```python
from build123d import *

# Parameters (mm, degrees)
BOSS_EXTRUDE5_DEPTH = 3
CUT_EXTRUDE1_DEPTH  = 9


with BuildPart() as part:
    # Sketch3 → Boss-Extrude5 (new body)
    with BuildSketch(Plane.XY):
        Polygon((-125, 125), (-125, -125), (25, -125), (35, -135), (125, -135), (125, -125), (125, 125), (125, 130), (95, 130), (90, 125), (20, 125), (15, 130), (-15, 130), (-20, 125), (-90, 125), (-95, 130), (-125, 130), align=None)
    extrude(amount=-BOSS_EXTRUDE5_DEPTH)

    # Sketch4 → Cut-Extrude1 (cut)
    with BuildSketch(Plane.XY):
        Polygon((34.899494937, -132.071067812), (41.970562748, -125), (27.828427125, -125), align=None)
        Polygon((37.727922061, -132.071067812), (46.213203436, -132.071067812), (41.970562748, -127.828427125), align=None)
    extrude(amount=-CUT_EXTRUDE1_DEPTH, mode=Mode.SUBTRACT)


solid = part.part
```
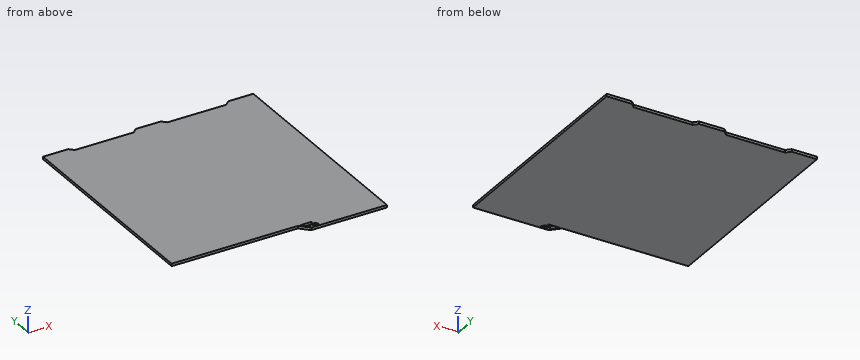
Geometry check sheet. Reference: the model listing, model coordinates, mm. Coordinates: 2 decimals unless noted, no trailing zeros. Loops run counter-clockwise (first coordinate to the right, second up) from the corner with the lowest first, then second, coordinate; pieces in that order, holes last.
Item 1: Sectioned sample at A-A, the plane z = -1. Record the boundary of the cut face in (x, y).
Item 2: Sectioned sample at B-B, the plane x = -103. Record the boundary of the cut face in (y, z), then the cut area to 3 significant figures.
Item 3: Go/stop test with a flat-tipped pin: pin 1 Ø0.9 at (x, z) = (63, -1.5) entering from +Y. Record where the tip stops, or that it passes through.
Item 4: Thickness scan on line 1 (Y direction, x = 12, z = -2.65); line 2 (Y direction, x = 53, z = -0.55). Record the ranges inside material, lowest first.
Item 5: Sectioned sample at C-C, the plane x = 77. Record the boundary of the cut face in (y, z).
Check result:
1. outline: (-125, -125) - (25, -125) - (35, -135) - (125, -135) - (125, 130) - (95, 130) - (90, 125) - (20, 125) - (15, 130) - (-15, 130) - (-20, 125) - (-90, 125) - (-95, 130) - (-125, 130) - close; hole (27.83, -125) - (34.9, -132.07) - (41.97, -125) - close; hole (37.73, -132.07) - (46.21, -132.07) - (41.97, -127.83) - close
2. outline: (-125, -3) - (130, -3) - (130, 0) - (-125, 0) - close
2. area: 765 mm2
3. pin 1: stops at y = 125
4. line 1: y = -125 to 130
4. line 2: y = -135 to 125
5. outline: (-135, -3) - (125, -3) - (125, 0) - (-135, 0) - close
